from build123d import *

# Parameters (mm, degrees)
F0_R     = 38.1
F1_DEPTH = 203.2
F2_R     = 38.1
F2_R_2   = 31.75
F3_DEPTH = 139.7
F4_R     = 31.75
F4_R_2   = 22.86
F5_DEPTH = 88.9
F6_R     = 31.75
F6_R_2   = 15.875
F7_DEPTH = 50.8
F8_R     = 15.875
F8_R_2   = 11.43
F9_DEPTH = 25.4


with BuildPart() as f1:
    # F0 (on Right) → F1 (new body)
    with BuildSketch(Plane.YZ):
        Circle(F0_R)
    extrude(amount=F1_DEPTH)

    # F2 (on face) → F3 (cut)
    with BuildSketch(Plane(origin=(0, 0, 0), x_dir=(0, -1, 0), z_dir=(-1, 0, 0))):
        Circle(F2_R)
        Circle(F2_R_2, mode=Mode.SUBTRACT)
    extrude(amount=-F3_DEPTH, mode=Mode.SUBTRACT)

    # F4 (on face) → F5 (cut)
    with BuildSketch(Plane(origin=(0, 0, 0), x_dir=(0, -1, 0), z_dir=(-1, 0, 0))):
        Circle(F4_R)
        Circle(F4_R_2, mode=Mode.SUBTRACT)
    extrude(amount=-F5_DEPTH, mode=Mode.SUBTRACT)

    # F6 (on face) → F7 (cut)
    with BuildSketch(Plane(origin=(0, 0, 0), x_dir=(0, -1, 0), z_dir=(-1, 0, 0))):
        Circle(F6_R)
        Circle(F6_R_2, mode=Mode.SUBTRACT)
    extrude(amount=-F7_DEPTH, mode=Mode.SUBTRACT)

    # F8 (on face) → F9 (cut)
    with BuildSketch(Plane(origin=(0, 0, 0), x_dir=(0, -1, 0), z_dir=(-1, 0, 0))):
        Circle(F8_R)
        Circle(F8_R_2, mode=Mode.SUBTRACT)
    extrude(amount=-F9_DEPTH, mode=Mode.SUBTRACT)


solid = f1.part
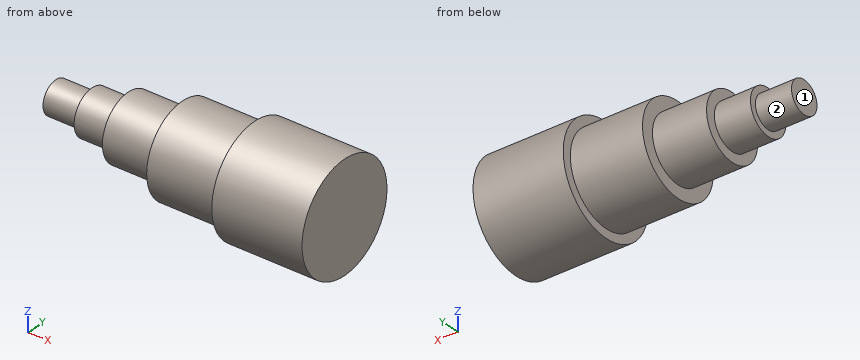
Geometry: final body of the model. Coordinates: model frame, mm. Face numbers are marked on the shaded views. A direction names the side the tool comes from. Round coordinates to 2 decimals unless told otherwise and drop trailing zeros. Loops run counter-clockwise (first coordinate to the right, second up) from the corner with the lowest first, then second, coordinate; pieces in that order, holes last.
Q1. Section C-C on x = 187. Return loops of the section in (y, z).
Q2. Section D-D on z = -18.5. Return loops of the section in (x, y).
Q3. Access query for the marked faces 1 and 2. Directions: +Z, -Z, +X, -X, +Y, -Y. A direction counts if a zero-diameter tool reaches every point of the face in a straight line with its end or side. Return the directions, or none.
Q4. Pin query (flat end, axial travel): P1, Ø6, axis at x = 105.5, z = -1, coming from the -Y side; P2, Ø3, axis at x = 167.5, z = -16.5, coming from the -Y side; P3, Ø2, axis at y = 14.5, z = 25, coming from the -X side. Return the tip coordinate at first contact, or that it passes through.
Q5. Section A-A on z = 0. Return loops of the section in (x, y) (3 decimals).
Q6. Material intervals for L1, parallel to X at y = -28.5, z = 4; L2, parallel to X at y = -16.5, z = 0.5; L3, parallel to Z at x = 113, y = 1.5, sorted ascending.
Evaluation:
1. outline: circle Ø76.2 at (0, 0)
2. outline: (50.8, -13.43) - (88.9, -13.43) - (88.9, -25.8) - (139.7, -25.8) - (139.7, -33.31) - (203.2, -33.31) - (203.2, 33.31) - (139.7, 33.31) - (139.7, 25.8) - (88.9, 25.8) - (88.9, 13.43) - (50.8, 13.43) - close
3. face 1: +Z, -Z, -X, +Y, -Y
3. face 2: -X
4. P1: stops at y = -31.75
4. P2: stops at y = -35.02
4. P3: stops at x = 88.9
5. outline: (0, -11.43) - (25.4, -11.43) - (25.4, -15.875) - (50.8, -15.875) - (50.8, -22.86) - (88.9, -22.86) - (88.9, -31.75) - (139.7, -31.75) - (139.7, -38.1) - (203.2, -38.1) - (203.2, 38.1) - (139.7, 38.1) - (139.7, 31.75) - (88.9, 31.75) - (88.9, 22.86) - (50.8, 22.86) - (50.8, 15.875) - (25.4, 15.875) - (25.4, 11.43) - (0, 11.43) - close
6. L1: x = 88.9 to 203.2
6. L2: x = 50.8 to 203.2
6. L3: z = -31.71 to 31.71
